Work out the finished part from the listing and answer in its coordinate system (mm). A direction names the side the tool comes from. Round coordinates to 2 decimals unless told otherwise and drop trailing zeros. Write each loop counter-clockwise with the first axis right and the second up, starting at its lowest first coordinate (ties: lowest second). Pieces come first, ordered by that corner, then holes.
1. Flat-ended cylindrical pins translate along their axes: pin 1 Ø0.6 at (y, z) = (-436, 6.5) entering from -X; pin 2 Ø6 at (y, z) = (-431.5, 3) entering from +X; pin 3 Ø3 at (y, z) = (-433.5, 6) entering from +X. Find the tip coordinate at first contact, or state that the pin passes through.
2. Find section C-C (x = 577.5). Write down the section's boundary in (y, z), and give its area (3 significant figures).
3. Find section B-B (y = -427.5). Write down the section's boundary in (x, z).
4. Determine the mould class of faces 1 (the face through (619, -446.296, 5)), 2 (the face through (575, -415.296, 5)), 3 (the face through (681.484, -440.593, 4.93)), 4 (the face through (559.555, -405.909, 4.93)) for opening direction X: pulls with the +X half, pulls with the -X half, needs draft (parallel to the pull), parting line crosses it, or undercut.
5. A tool of negligible diameter and unlimited length cuts with its end or side. For faces 5 (the face through (619, -428, 0)), 6 (the face through (619, -426.296, 5)), 7 (the face through (681.492, -409, 5)), from which of +Z, -Z, +X, -X, +Y, -Y can it reach the whole face along a straight path? Write none if from no direction.
6. Straight lines are drawn through the part: probe 1 along X at (y, z) = (-422.5, 6.5); probe 2 along X at (y, z) = (-408.5, 9); probe 3 along X at (y, z) = (-426.5, 2.5). For each, find the intervals that lie inside material, in ascending order.
7. Find section A-A (y = -422.5). Write down the section's boundary in (x, z), and give its area (3 significant figures).
8. Find section D-D (z = 1.5). Count the separate pieces of the cut face and the enclosed holes in it, and give its area (3 significant figures).
```python
from build123d import *

# Parameters (mm, degrees)
DODANIE_WYCI_GNI_CIE1_DEPTH = 10
SZKIC2_R                    = 1.55
WYTNIJ_WYCI_GNI_CIE1_DEPTH  = 10
WYTNIJ_WYCI_GNI_CIE2_DEPTH  = 10
DODANIE_WYCI_GNI_CIE2_DEPTH = 10


with BuildPart() as part:
    # Szkic1 → Dodanie-wyciągnięcie1 (new body)
    with BuildSketch(Plane.XY):
        with BuildLine():
            Line((587.414080321, -426.296177349), (650.882642176, -426.296177349))
            ThreePointArc((650.882642176, -426.296177349), (651.591558731, -426.002534497), (651.885201582, -425.293617942))
            Line((651.885201582, -425.293617942), (651.885201582, -419.296173179))
            ThreePointArc((651.885201582, -419.296173179), (653.056774457, -416.467746055), (655.885201582, -415.296173179))
            Line((655.885201582, -415.296173179), (672.570535687, -415.296173179))
            add(Edge.make_bspline(
                [(672.570535687, -415.296173179), (680.339252511, -414.463378733), (681.492424358, -410.309612352)],
                knots=[0, 0, 0, 1, 1, 1], degree=2))
            Line((681.492424358, -410.309612352), (681.492424358, -407.696232794))
            ThreePointArc((681.492424358, -407.696232794), (680.760191311, -405.928465841), (678.992424358, -405.196232794))
            ThreePointArc((678.992424358, -405.196232794), (676.992424358, -403.196232794), (678.992424358, -401.196232794))
            Line((678.992424358, -401.196232794), (680.992424358, -401.196232794))
            ThreePointArc((680.992424358, -401.196232794), (685.588618435, -403.100038717), (687.492424358, -407.696232794))
            Line((687.492424358, -407.696232794), (687.492424358, -412.4992576))
            Line((687.492424358, -412.4992576), (687.497764867, -419.296173358))
            ThreePointArc((687.497764867, -419.296173358), (681.63990049, -433.438308981), (667.497764867, -439.296173358))
            Line((667.497764867, -439.296173358), (572.803105375, -439.296173358))
            ThreePointArc((572.803105375, -439.296173358), (558.660969752, -433.438308981), (552.803105375, -419.296173358))
            Line((552.803105375, -419.296173358), (552.803105375, -407.696232794))
            ThreePointArc((552.803105375, -407.696232794), (554.706911183, -403.100038993), (559.303104985, -401.196233185))
            Line((559.303104985, -401.196233185), (561.303104985, -401.196232404))
            ThreePointArc((561.303104985, -401.196232404), (563.303105554, -403.196232208), (561.303105749, -405.196232777))
            ThreePointArc((561.303105749, -405.196232777), (559.535338555, -405.928465692), (558.803105376, -407.696232777))
            Line((558.803105376, -407.696232777), (558.803105375, -410.309612352))
            add(Edge.make_bspline(
                [(567.724994046, -415.296173179), (559.956277223, -414.463378733), (558.803105375, -410.309612352)],
                knots=[0, 0, 0, 1, 1, 1], degree=2))
            Line((567.724994046, -415.296173179), (582.555068068, -415.296173179))
            ThreePointArc((582.555068068, -415.296173179), (585.383495193, -416.467746055), (586.555068068, -419.296173179))
            Line((586.555068068, -419.296173179), (586.555068068, -425.296173358))
            ThreePointArc((586.555068068, -425.296173358), (586.777466587, -425.974082616), (587.414080321, -426.296177349))
        make_face()
    extrude(amount=DODANIE_WYCI_GNI_CIE1_DEPTH)

    # Szkic2 → Wytnij-wyciągnięcie1 (cut)
    with BuildSketch(Plane.XY.offset(10)):
        with Locations((657.507953751, -432.275447831)):
            Circle(SZKIC2_R)
        with Locations((582.803105375, -432.296173587)):
            Circle(SZKIC2_R)
    extrude(amount=-WYTNIJ_WYCI_GNI_CIE1_DEPTH, mode=Mode.SUBTRACT)

    # Szkic3 → Wytnij-wyciągnięcie2 (cut)
    with BuildSketch(Plane(origin=(0, 0, 0), x_dir=(-1, 0, 0), z_dir=(0, 0, -1))):
        Polygon((-600.699082892, -426.296174265), (-600.699082892, -433.796174265), (-602.074082892, -433.796174265), (-602.074082892, -435.796174265), (-600.699082892, -435.796174265), (-600.699082892, -436.296174265), (-597.599082892, -436.296174265), (-597.599082892, -435.796174265), (-596.224082892, -435.796174265), (-596.224082892, -433.796174265), (-597.599082892, -433.796174265), (-597.599082892, -426.296174265), align=None)
        Polygon((-640.699082892, -426.296174265), (-640.699082892, -433.796174265), (-642.074082892, -433.796174265), (-642.074082892, -435.796174265), (-640.699082892, -435.796174265), (-640.699082892, -436.296174265), (-637.599082892, -436.296174265), (-637.599082892, -435.796174265), (-636.224082892, -435.796174265), (-636.224082892, -433.796174265), (-637.599082892, -433.796174265), (-637.599082892, -426.296174265), align=None)
    extrude(amount=-WYTNIJ_WYCI_GNI_CIE2_DEPTH, mode=Mode.SUBTRACT)

    # Szkic4 → Dodanie-wyciągnięcie2 (add)
    with BuildSketch(Plane(origin=(0, 0, 0), x_dir=(-1, 0, 0), z_dir=(0, 0, -1))):
        with BuildLine():
            Line((-572.80310596, -446.29617968), (-667.497765451, -446.296171767))
            ThreePointArc((-667.497765451, -446.296171767), (-681.639900798, -440.438306104), (-687.497764867, -426.296170096))
            Line((-687.497764867, -426.296170096), (-687.497764867, -419.296173358))
            ThreePointArc((-687.497764867, -419.296173358), (-681.63990049, -433.438308981), (-667.497764867, -439.296173358))
            Line((-667.497764867, -439.296173358), (-572.803105375, -439.296173358))
            ThreePointArc((-572.803105375, -439.296173358), (-558.660969752, -433.438308981), (-552.803105375, -419.296173358))
            Line((-552.803105375, -419.296173358), (-552.803105375, -426.296181351))
            ThreePointArc((-552.803105375, -426.296181351), (-558.660970549, -440.438316101), (-572.80310596, -446.29617968))
        make_face()
    extrude(amount=-DODANIE_WYCI_GNI_CIE2_DEPTH)


solid = part.part
```
Worked answers:
1. pin 1: stops at x = 555.15
1. pin 2: stops at x = 687.38
1. pin 3: stops at x = 686.67
2. outline: (-446.3, 0) - (-415.3, 0) - (-415.3, 10) - (-446.3, 10) - close
2. area: 310 mm2
3. outline: (552.84, 0) - (597.6, 0) - (597.6, 10) - (552.84, 10) - close; (600.7, 0) - (637.6, 0) - (637.6, 10) - (600.7, 10) - close; (640.7, 0) - (687.46, 0) - (687.46, 10) - (640.7, 10) - close
4. face 1: needs draft
4. face 2: undercut
4. face 3: pulls with the +X half
4. face 4: undercut
5. face 5: -Z, +X, -X, +Y, -Y
5. face 6: +Z, -Z, +Y
5. face 7: +Z, -Z
6. probe 1: x = 552.8 to 586.56, 651.89 to 687.5
6. probe 2: x = 552.8 to 558.8, 681.49 to 687.49
6. probe 3: x = 552.8 to 597.6, 600.7 to 637.6, 640.7 to 687.5
7. outline: (552.8, 0) - (586.56, 0) - (586.56, 10) - (552.8, 10) - close; (651.89, 0) - (687.5, 0) - (687.5, 10) - (651.89, 10) - close
7. area: 694 mm2
8. separate pieces: 1
8. enclosed holes: 2
8. area: 3,400 mm2
